from build123d import *

# Parameters (mm, degrees)
SKETCH_R        = 11
PAD_DEPTH       = 7
PAD001_DEPTH    = 5
SKETCH002_R     = 2
POCKET_DEPTH    = 9
POCKET002_DEPTH = 20
FILLET_R        = 30
FILLET001_R     = 5
SKETCH005_W     = 10
SKETCH005_H     = 22
POCKET003_DEPTH = 15
CHAMFER_SIZE    = 4
FILLET002_R     = 0.8
FILLET003_R     = 1.5
FILLET004_R     = 1.5
FILLET005_R     = 1.5


with BuildPart() as part:
    # Sketch → Pad (new body)
    with BuildSketch(Plane.XY):
        with BuildLine():
            Line((-15, -48), (15, -48))
            Line((15, -48), (15, -14.696938))
            ThreePointArc((15, -14.696938), (24.166051, 8.774235), (-0.998465, 7.48598))
            Line((-45, -48), (-0.998465, 7.48598))
            Line((-45, -48), (-15, -48))
        make_face()
        with Locations((12, 0)):
            Circle(SKETCH_R, mode=Mode.SUBTRACT)
    extrude(amount=PAD_DEPTH)

    # Sketch001 (on Face6 of Pad) → Pad001 (join)
    with BuildSketch(Plane.XY.offset(7)):
        Polygon((-45, -48), (-40.385913, -40), (15, -40), (15, -48), align=None)
    extrude(amount=PAD001_DEPTH)

    # Sketch002 (on Face11 of Pad001) → Pocket (cut)
    with BuildSketch(Plane.XZ.offset(48)):
        with Locations((-20, 4)):
            Circle(SKETCH002_R)
        with Locations((4, 4)):
            Circle(SKETCH002_R)
    extrude(amount=-POCKET_DEPTH, mode=Mode.SUBTRACT)

    # Sketch004 → Pocket002 (cut)
    with BuildSketch(Plane.XY.offset(12)):
        Polygon((-27.492516, -50.55183), (-27.492516, -40), (-12.942459, -40), (-12.942459, 0), (-27.492525, 0), (-27.492525, 11.934225), (-46.836239, 11.934225), (-46.836239, -50.55183), align=None)
    extrude(amount=-POCKET002_DEPTH, mode=Mode.SUBTRACT)

    # Fillet
    fillet_edges = [part.edges().sort_by_distance(p)[0] for p in [
        (-12.942459, -7.575408, 3.5),
    ]]
    fillet(fillet_edges, radius=FILLET_R)

    # Fillet001
    fillet001_edges = [part.edges().sort_by_distance(p)[0] for p in [
        (15, -14.696938, 3.5),
    ]]
    fillet(fillet001_edges, radius=FILLET001_R)

    # Sketch005 (on Face12 of Fillet001) → Pocket003 (cut)
    with BuildSketch(Plane.XY.offset(7)):
        with Locations((3.99969, -29.002266)):
            Rectangle(SKETCH005_W, SKETCH005_H)
    extrude(amount=-POCKET003_DEPTH, mode=Mode.SUBTRACT)

    # Chamfer
    chamfer_edges = [part.edges().sort_by_distance(p)[0] for p in [
        (-6.971384, -40, 7),
        (11.999845, -40, 7),
    ]]
    chamfer(chamfer_edges, length=CHAMFER_SIZE)

    # Fillet002
    fillet002_edges = [part.edges().sort_by_distance(p)[0] for p in [
        (-6.246258, -40, 12),
    ]]
    fillet(fillet002_edges, radius=FILLET002_R)

    # Fillet003
    fillet003_edges = [part.edges().sort_by_distance(p)[0] for p in [
        (-27.492516, -44.4, 12),
        (-27.492516, -40.234315, 11.765685),
        (-27.492516, -40, 5.6),
    ]]
    fillet(fillet003_edges, radius=FILLET003_R)

    # Fillet004
    fillet004_edges = [part.edges().sort_by_distance(p)[0] for p in [
        (-12.942459, -38, 9),
        (-12.942459, -27.01348, 7),
        (-11.272446, -8.157216, 7),
        (-3.7234, 4.049834, 7),
        (23.17865, 10.001889, 7),
        (15.8167, -15.59169, 7),
        (15, -27.165151, 7),
        (15, -38, 9),
        (15, -40, 11.1),
        (15, -40.234315, 11.765685),
        (15, -44.4, 12),
    ]]
    fillet(fillet004_edges, radius=FILLET004_R)

    # Fillet005
    fillet005_edges = [part.edges().sort_by_distance(p)[0] for p in [
        (-1.00031, -38, 9),
        (-1.00031, -27.001133, 7),
        (3.99969, -18.002266, 7),
        (8.99969, -27.001133, 7),
        (8.99969, -38, 9),
    ]]
    fillet(fillet005_edges, radius=FILLET005_R)


solid = part.part
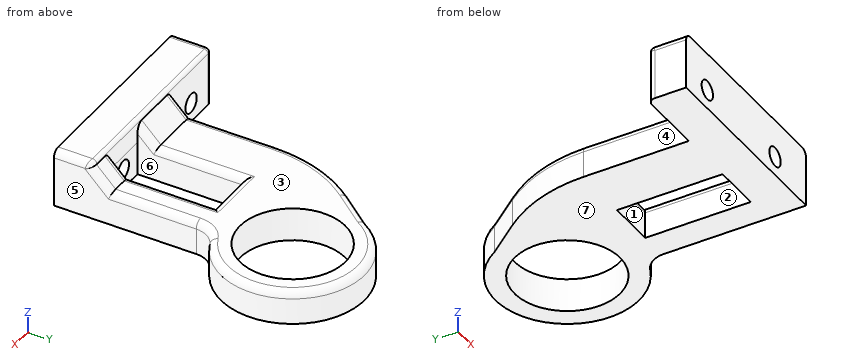
Verification items for the finished model (mm, model axes). Face numbers are marked on the shaded views. A direction names the side the tool comes from. Coordinates: 2 decimals unless noted, no trailing zeros. Loops run counter-clockwise (first coordinate to the right, second up) from the corner with the lowest first, then second, coordinate; pieces in that order, holes last. Notation, with made-up numbers: (63.25, -35.75) -> (79.25, -35.75) arc R29 cw to (79.25, -11.75) -> close; hole circle Ø10 at (-39, 75). An arc over 180 degrees is marked (long way). Answer as a JSON object with one key per item and string values. Group by question number.
Item 1: Scan lines: probe 1 along Y at (x, z) = (12, 1.5); probe 2 along Z at (x, y) = (-20, -41); probe 3 along X at (y, z) = (9.5, 6). Record each from-to range of solid material in increasing order.
Item 2: Sectioned sample at C-C on z = 4. Record the boundary of the cut face in (x, y), plus the area to 3 significant figures.
Item 3: Depth check by flat-ended pin: pin 1 (3 mm diameter, centred on y = 8.5, z = 1.5, fed in from -X); pin 2 (5.5 mm diameter, centred on x = -15, z = 8, fed in from +Y); pin 3 (7 mm diameter, centred on y = -33, z = 5.5, fed in from +X). Enter the tip coordinate at first touch or a pass-through.
Item 4: Tool access check on the marked faces 5, 6 and 7. Record the directions out of +Z, -Z, +X, -X, +Y, -Y that give a thin tool (end or side, any length) a straight path to the whole face; none if there is none.
Item 5: Sectioned sample at B-B on y = -32. Record the boundary of the cut face in (x, z).
Item 6: Sectioned sample at D-D on x = -14. Record the boundary of the cut face in (y, z).
Item 7: Sectioned sample at A-A on x = -20. Record the boundary of the cut face in (y, z).
Item 8: Mould release check, pull along X, two halves, no side actions. Record for the marked faces 1, 2, 3 and 4: +X half, -X half, draft (parallel to the pull), parting line (faces both ways), or undercut.
Evaluation:
{
 "1": {"probe 1": "y = -48 to -11, 11 to 15", "probe 2": "z = 0 to 2, 6 to 12", "probe 3": "x = 0.5 to 6.45, 17.55 to 23.5"},
 "2": {"outline": "(-27.49, -48) -> (-22, -48) -> (-22, -40) -> (-25.99, -40) arc R1.5 ccw to (-27.49, -41.5) -> close; (-18, -48) -> (2, -48) -> (2, -40) -> (-1, -40) -> (-1, -18) -> (9, -18) -> (9, -40) -> (6, -40) -> (6, -48) -> (15, -48) -> (15, -18.33) arc R5 cw to (18, -13.75) arc R15 ccw (long way) to (-1, 7.49) -> (-6.45, 0.61) arc R30 ccw to (-12.94, -18.03) -> (-12.94, -40) -> (-18, -40) -> close; hole circle Ø22 at (12, 0)", "area": "1,260 mm²"},
 "3": {"pin 1": "stops at x = -1.38", "pin 2": "stops at y = -36.43", "pin 3": "stops at x = 15"},
 "4": {"face 5": "+Z, -Z, +X, -Y", "face 6": "+Z, -Z", "face 7": "-Z, +X, -X, +Y, -Y"},
 "5": {"outline": "(-12.94, 0) -> (-1, 0) -> (-1, 5.5) arc R1.5 ccw to (-2.5, 7) -> (-11.44, 7) arc R1.5 ccw to (-12.94, 5.5) -> close; (9, 0) -> (15, 0) -> (15, 5.5) arc R1.5 ccw to (13.5, 7) -> (10.5, 7) arc R1.5 ccw to (9, 5.5) -> close"},
 "6": {"outline": "(-48, 0) -> (-40, 0) -> (-40, 11.2) arc R0.8 ccw to (-40.8, 12) -> (-48, 12) -> close"},
 "7": {"outline": "(-48, 0) -> (-40, 0) -> (-40, 2) -> (-48, 2) -> close; (-48, 6) -> (-40, 6) -> (-40, 11.2) arc R0.8 ccw to (-40.8, 12) -> (-48, 12) -> close"},
 "8": {"face 1": "undercut", "face 2": "undercut", "face 3": "draft", "face 4": "-X half"}
}
